Part print with two shaded views. Sizes in mm from the minimum x, y, z corner. A direction names the side the tool comes from. Round coordinates to 2 decimals unless told otherwise and drop trailing zeros. Write each loop counter-clockwise with the first axis right and the second up, starting at its lowest first coordinate (ties: lowest second). Pieces come first, ordered by that corner, then holes. Notation, with made-up numbers: M 78,70 L 129,70 A21 cw 129,92 Z; hole C 15.25,17.25 d7. An arc over 180 degrees is marked long. Use one line per item in the form item = value. Start each with the question number.
Item 1: Cut at A-A, the plane z = 25.4. Give the cut face in (x, y) (1 decimal).
Item 2: Flat gauge pins, fed straight in: pin 1 Ø3 at (x, z) = (33.5, 37.5) entering from -Y; pin 2 Ø6 at (x, z) = (36.5, 9) entering from +Y (3 decimals); pin 3 Ø1 at (x, y) = (35.5, 15) entering from +Z. Where does each tip first touch, or does it go through?
Item 3: Cut at C-C, the plane y = 22.5. Give the cut face in (x, z).
Item 4: Probe L1, parallel to Y at x = 27, z = 39.5 (3 decimals); L2, parallel to Z at x = 29.5, y = 43; L3, parallel to Z at x = 32.5, y = 14. List the from-to ranges inside material, lowest first.
Item 5: Which spindle directions (+Z, -Z, +X, -X, +Y, -Y) get a long thin tool onto all of the face, cutting with end or side? Do the marked faces 1, 2 and 3. Say none if no direction does.
Item 6: Cut at D-D, the plane y = 9.5. Give the cut face in (x, z) (1 decimal).
Item 7: Cut at B-B, the plane x = 26. Give the cut face in (y, z) (3 decimals), then the cut area to 3 significant figures.
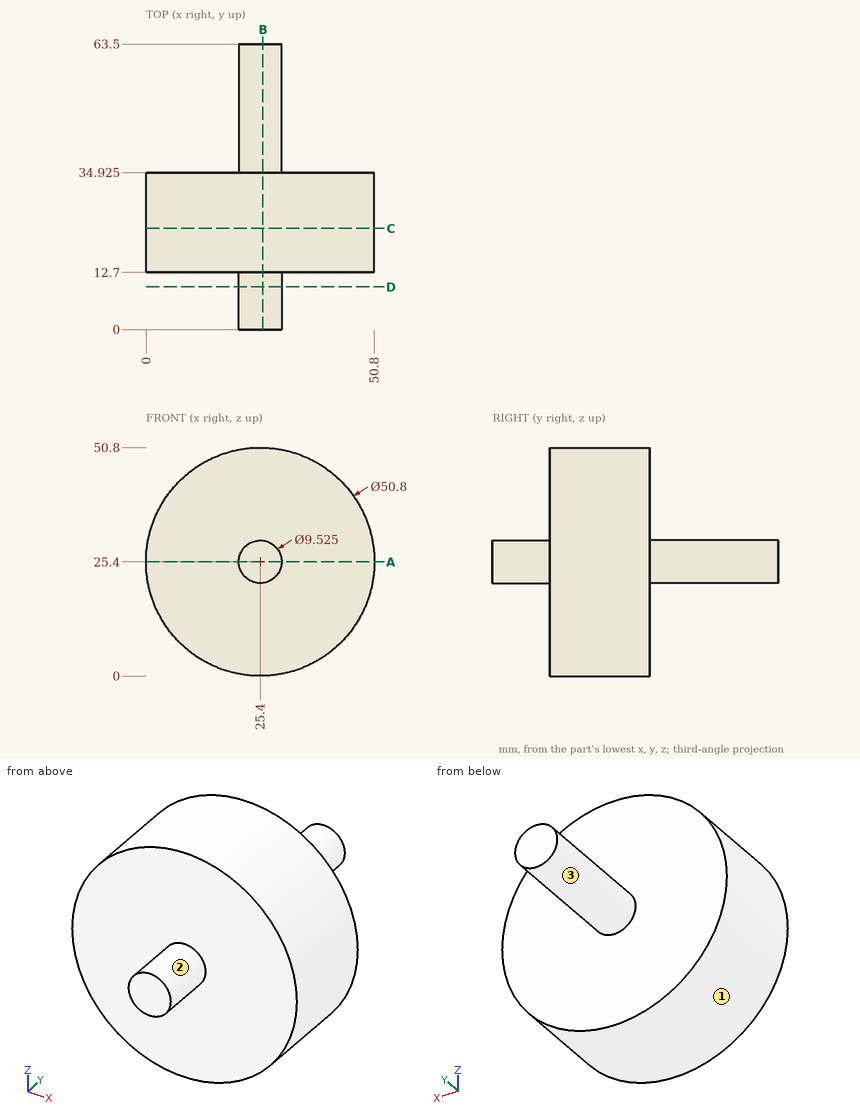
Model answer:
q1.outline = M 0,12.7 L 20.6,12.7 L 20.6,0 L 30.2,0 L 30.2,12.7 L 50.8,12.7 L 50.8,34.9 L 30.2,34.9 L 30.2,63.5 L 20.6,63.5 L 20.6,34.9 L 0,34.9 Z
q2.pin_1 = 12.7
q2.pin_2 = 34.925
q2.pin_3 = 48.92
q3.outline = C 25.4,25.4 d50.8
q4.L1 = 12.7 to 34.925
q4.L2 = 22.98 to 27.82
q4.L3 = 1.01 to 49.79
q5.face_1 = +Y, -Y
q5.face_2 = -Y
q5.face_3 = +Y
q6.outline = C 25.4,25.4 d9.5
q7.outline = M 0,20.675 L 12.7,20.675 L 12.7,0.007 L 34.925,0.007 L 34.925,20.675 L 63.5,20.675 L 63.5,30.125 L 34.925,30.125 L 34.925,50.793 L 12.7,50.793 L 12.7,30.125 L 0,30.125 Z
q7.area = 1,520 mm²
